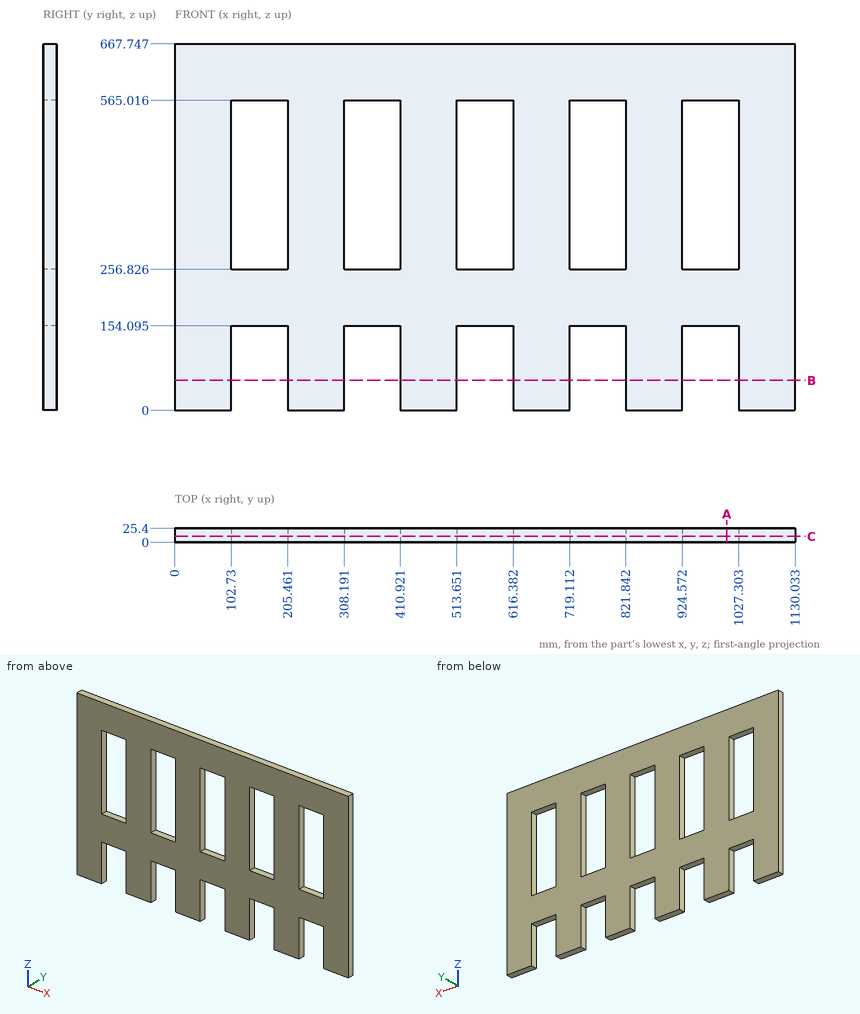
Input: dimensioned drawing with shaded views. Units: mm. Origin: part minimum x, y, z. Give positions to 0.01 mm unless a question says otherwise; leave off trailing zeros. Write each loop counter-clockwise with the first axis right and the second up, starting at its lowest first coordinate (ties: lowest second). Pieces come first, ordered by that corner, then holes. Notation, with made-up numbers: M -5.5,72 L 14.5,72 A35 ccw 14.5,107 Z; hole C 2,52.25 d8. An arc over 180 degrees is marked long. Return JSON: item names as keys, results as strings. Group by question number.
1) Pin query (flat end, axial travel): P1, Ø12.5, axis at x = 554.5, y = 9, coming from the -Z side (1 decimal). Return the tip coordinate at first contact, or that it passes through.
2) Cut plane C-C, the plane y = 11. Give the number of separate pieces and of enclosed holes in the cut face, plus the area to 3 significant figures.
3) Cut plane A-A, the plane x = 1006. Output: boundary loops of the cut face in (y, z) (1 decimal).
4) Cut plane B-B, the plane z = 54.5. Output: boundary loops of the cut face in (x, y), plus the area to 3 significant figures.
5) Material intervals for line 1 along X through (y, z) = (6.5, 526.5); line 2 along Z through (x, y) = (817, 14.5) (1 decimal), sorted ascending. Write a range as [from, to].
Recorded:
{
 "1": {"P1": "stops at z = 154.1"},
 "2": {"separate pieces": "1", "enclosed holes": "5", "area": "517,000 mm²"},
 "3": {"outline": "M 0,154.1 L 25.4,154.1 L 25.4,256.8 L 0,256.8 Z; M 0,565 L 25.4,565 L 25.4,667.7 L 0,667.7 Z"},
 "4": {"outline": "M 0,0 L 102.73,0 L 102.73,25.4 L 0,25.4 Z; M 205.46,0 L 308.19,0 L 308.19,25.4 L 205.46,25.4 Z; M 410.92,0 L 513.65,0 L 513.65,25.4 L 410.92,25.4 Z; M 616.38,0 L 719.11,0 L 719.11,25.4 L 616.38,25.4 Z; M 821.84,0 L 924.57,0 L 924.57,25.4 L 821.84,25.4 Z; M 1027.3,0 L 1130.03,0 L 1130.03,25.4 L 1027.3,25.4 Z", "area": "15,700 mm²"},
 "5": {"line 1": "x = [0, 102.73], [205.46, 308.19], [410.92, 513.65], [616.38, 719.11], [821.84, 924.57], [1027.3, 1130.03]", "line 2": "z = [154.1, 256.8], [565, 667.7]"}
}
